Design review of the part built by this model. Coordinates are the model's own, in mm. Coordinates: 2 decimals unless noted, no trailing zeros. Loops run counter-clockwise (first coordinate to the right, second up) from the corner with the lowest first, then second, coordinate; pieces in that order, holes last. Notation, with made-up numbers: (73, 53) -> (129, 53) arc R17 cw to (129, 66) -> close; hole circle Ø11 at (-40, -20). An arc over 180 degrees is marked (long way). Use CSV: the item, a comma, the result in double quotes.
```python
from build123d import *

# Parameters (mm, degrees)
F0_R     = 25
F1_DEPTH = 200
F2_SIZE  = 50


with BuildPart() as f1:
    # F0 (on Front) → F1 (new body)
    with BuildSketch(Plane.XZ):
        with BuildLine():
            ThreePointArc((100, 175), (92.67767, 192.67767), (75, 200))
            Line((75, 200), (-75, 200))
            ThreePointArc((-75, 200), (-92.67767, 192.67767), (-100, 175))
            Line((-100, 175), (-100, -200))
            Line((-100, -200), (100, -200))
            Line((100, -200), (100, 175))
        make_face()
        Circle(F0_R, mode=Mode.SUBTRACT)
    extrude(amount=F1_DEPTH)

    # F2
    f2_edges = [f1.edges().sort_by_distance(p)[0] for p in [
        (100, -100, -200),
        (-100, -100, -200),
    ]]
    chamfer(f2_edges, length=F2_SIZE)


solid = f1.part
```
Item 1: Add section D-D (x = -65). Give the boundary of the cut face in (y, z), then the cut area to 3 significant figures.
Checked values:
outline,"(-200, -185) -> (0, -185) -> (0, 200) -> (-200, 200) -> close"
area,"77,000 mm^2"
Item 2: Add section A-A (z = 0). Give the boundary of the cut face in (x, y), then the cut area to 3 significant figures.
Checked values:
outline,"(-100, -200) -> (-25, -200) -> (-25, 0) -> (-100, 0) -> close; (25, -200) -> (100, -200) -> (100, 0) -> (25, 0) -> close"
area,"30,000 mm^2"
Item 3: Draft analysis for pull direction X (two halves, no side actions). For faces 1 (the face through (-1, -99, -200)), 2 (the face through (-100, -99, 15)), 3 (the face through (92.871, -98.6, 192.482)), 4 (the face through (23.846, -98.6, 7.509)), state which applies: pulls with the +X half, pulls with the -X half, needs draft (parallel to the pull), parting line crosses it, or undercut.
Checked values:
face 1,"needs draft"
face 2,"pulls with the -X half"
face 3,"pulls with the +X half"
face 4,"undercut"
Item 4: To check wall thickness, follow line 1 along Z through (x, y) = (0, -95); line 2 along X through (y, z) = (-103, 176.5); line 3 along Z through (x, y) = (17, -40.5). State the ranges of each line that lie inside material, in increasing order.
Checked values:
line 1,"-200 to -25, 25 to 200"
line 2,"-99.95 to 99.95"
line 3,"-200 to -18.33, 18.33 to 200"
Item 5: Clearance check with a flat-ended pin moving along its axis: pin 1 (8 mm diameter, centred on x = 36.5, z = -3.5, fed in from +Y). State where the tip first meets the part, or that it passes through.
Checked values:
pin 1,"y = 0"
Item 6: Add section C-C (x = -5.5). Give the boundary of the cut face in (y, z), then the cut area to 3 significant figures.
Checked values:
outline,"(-200, -200) -> (0, -200) -> (0, -24.39) -> (-200, -24.39) -> close; (-200, 24.39) -> (0, 24.39) -> (0, 200) -> (-200, 200) -> close"
area,"70,200 mm^2"
Item 7: Add section B-B (y = -117). Give the boundary of the cut face in (x, z).
Checked values:
outline,"(-100, -150) -> (-50, -200) -> (50, -200) -> (100, -150) -> (100, 175) arc R25 ccw to (75, 200) -> (-75, 200) arc R25 ccw to (-100, 175) -> close; hole circle Ø50 at (0, 0)"
